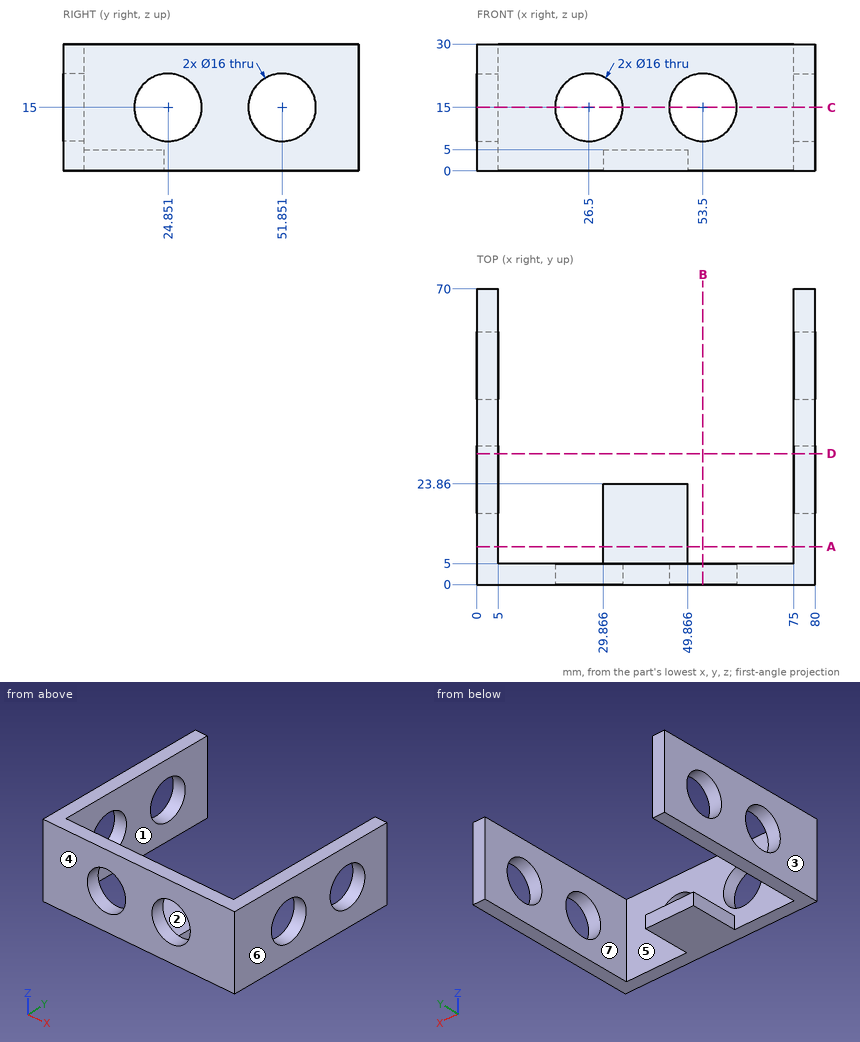
Verification items for this drawing (mm, ordinates from the low corner). A direction names the side the tool comes from. Give positions to 0.01 mm unless a question says otherwise; leave off trailing zeros. Loops run counter-clockwise (first coordinate to the right, second up) from the corner with the lowest first, then second, coordinate; pieces in that order, holes last.
(1) Release check for a two-part mould opening along X. For the marked faces 4, 5, 6 and 7 record: released by +X, released by -X, zero draft, split by the parting line, or undercut.
From the geometry:
face 4: zero draft
face 5: undercut
face 6: released by +X
face 7: undercut
(2) Thickness scan on L1, parallel to Y at x = 77.5, z = 15; L2, parallel to X at y = 20, z = 8; L3, parallel to X at y = 4.5, z = 15.5 (1 decimal). Record the ranges inside material, lowest first.
From the geometry:
L1: y = 0 to 16.85, 32.85 to 43.85, 59.85 to 70
L2: x = 0 to 5, 75 to 80
L3: x = 0 to 18.5, 34.5 to 45.5, 61.5 to 80
(3) Section check B-B on x = 53.5. Record the cut outline in (y, z), then the cut area to 3 significant figures.
From the geometry:
outline: (0, 0) - (5, 0) - (5, 7) - (0, 7) - close; (0, 23) - (5, 23) - (5, 30) - (0, 30) - close
area: 70.0 mm2
(4) Depth check by flat-ended pin: pin 1 Ø1.5 at (x, z) = (39, 2) entering from +Y; pin 2 Ø9.5 at (x, y) = (39.5, 12) entering from +Z. Enter the tip coordinate at first touch or a pass-through.
From the geometry:
pin 1: stops at y = 23.86
pin 2: stops at z = 5
(5) Section check D-D on y = 31. Record the cut outline in (x, z), then the cut area to 3 significant figures.
From the geometry:
outline: (0, 0) - (5, 0) - (5, 9.88) - (0, 9.88) - close; (0, 20.12) - (5, 20.12) - (5, 30) - (0, 30) - close; (75, 0) - (80, 0) - (80, 9.88) - (75, 9.88) - close; (75, 20.12) - (80, 20.12) - (80, 30) - (75, 30) - close
area: 198 mm2
(6) Section check A-A on y = 9. Record the cut outline in (x, z), then the cut area to 3 significant figures.
From the geometry:
outline: (0, 0) - (5, 0) - (5, 30) - (0, 30) - close; (29.87, 0) - (49.87, 0) - (49.87, 5) - (29.87, 5) - close; (75, 0) - (80, 0) - (80, 30) - (75, 30) - close
area: 400 mm2
(7) Section check C-C on z = 15. Count the separate pieces of the cut face and the enclosed holes in it, then the cut area to 3 significant figures.
From the geometry:
separate pieces: 7
enclosed holes: 0
area: 570 mm2
(8) Set-up check for the marked faces 1, 2 and 3: record each of +Z, -Z, +X, -X, +Y, -Y from which the full face is reachable in a straight line by a thin tool's end or side.
From the geometry:
face 1: +Z, -Z, +Y
face 2: +Z, +Y
face 3: +Z, -Z, -X, +Y, -Y
